Input: part model. Units: mm. Frame: model coordinates. A direction names the side the tool comes from. Round coordinates to 2 decimals unless told otherwise and drop trailing zeros. Loops run counter-clockwise (first coordinate to the right, second up) from the corner with the lowest first, then second, coordinate; pieces in that order, holes last. Notation, with made-up numbers: (18.5, -5.5) - (24.5, -5.5) arc R36 cw to (24.5, 33.5) - close; hole circle Ø4 at (50.5, -22.75). An arc over 180 degrees is marked (long way). One line per question, with ' | ' between items. Start each with the question number.
Item 1: First-contact query: pin 1 (13 mm diameter, centred on x = 11.5, y = 2.5, fed in from +Z); pin 2 (1.8 mm diameter, centred on x = -15.5, y = 17, fed in from -Z). Flat tips, straight axial feed; report the tip coordinate or a pass-through.
Item 2: Section B-B, the plane x = -15.5. Return loops of the section in (y, z), plus the area to 3 significant figures.
Item 3: Material intervals for line 1 along Y through (x, z) = (15.5, 2.5); line 2 along Y through (x, z) = (15.5, -1.8); line 3 along Y through (x, z) = (16, 33), sorted ascending.
Item 4: Set-up query: faces 4 (the face through (-17.07, -16.15, 2.46)), 5 (the face through (0, 0, 5)), 6 (the face through (-12.553, -15.63, -1.479)). Return all of +Z, -Z, +X, -X, +Y, -Y with unobstructed straight access to the full face (end or side cutting, diameter ignored); none if empty.
Item 5: Section D-D, the plane x = -3. Return loops of the section in (y, z).
Item 6: Section A-A, the plane y = -15.5. Return loops of the section in (x, z), plus the area to 3 significant figures.
Item 7: Section C-C, the plane z = 25. Return loops of the section in (x, y).
Item 8: Draft query along X for faces 1 (the face through (14, 14, 0)), 2 (the face through (26.5, 0, 0)), 3 (the face through (0, -24, 43)). Return one class per face: pulls with the +X half, pulls with the -X half, needs draft (parallel to the pull), parting line crosses it, or undercut.
```python
from build123d import *

# Parameters (mm, degrees)
SKETCH1_W           = 53
SKETCH1_H           = 43
BOSS_EXTRUDE1_DEPTH = 5
SKETCH2_W           = 53
SKETCH2_H           = 5
BOSS_EXTRUDE2_DEPTH = 43
SKETCH4_R           = 1.7
CUT_EXTRUDE1_DEPTH  = 58.039460025
SKETCH6_W           = 53
SKETCH6_H           = 53
SKETCH6_R           = 2.95
BOSS_EXTRUDE5_DEPTH = 3


with BuildPart() as part:
    # Sketch1 → Boss-Extrude1 (new body)
    with BuildSketch(Plane.XY):
        Rectangle(SKETCH1_W, SKETCH1_H)
    extrude(amount=BOSS_EXTRUDE1_DEPTH)

    # Sketch2 → Boss-Extrude2 (add)
    with BuildSketch(Plane(origin=(0, 0, 0), x_dir=(-1, 0, 0), z_dir=(0, 0, -1))):
        with Locations((0, -24)):
            Rectangle(SKETCH2_W, SKETCH2_H)
        with Locations((0, 24)):
            Rectangle(SKETCH2_W, SKETCH2_H)
    extrude(amount=-BOSS_EXTRUDE2_DEPTH)

    # Sketch4 → Cut-Extrude1 (cut, through all)
    with BuildSketch(Plane(origin=(0, 0, 0), x_dir=(-1, 0, 0), z_dir=(0, 0, -1))):
        with Locations((-15.5, 15.5)):
            Circle(SKETCH4_R)
        with Locations((15.5, 15.5)):
            Circle(SKETCH4_R)
        with Locations((-15.5, -15.5)):
            Circle(SKETCH4_R)
        with Locations((15.5, -15.5)):
            Circle(SKETCH4_R)
    extrude(amount=-CUT_EXTRUDE1_DEPTH, mode=Mode.SUBTRACT)

    # Sketch6 → Boss-Extrude5 (add)
    with BuildSketch(Plane.XY):
        Rectangle(SKETCH6_W, SKETCH6_H)
        with Locations((-15.5, 15.5)):
            Circle(SKETCH6_R, mode=Mode.SUBTRACT)
        with Locations(Location((15.5, 15.5, 0), (0, 0, 180))):
            Circle(SKETCH6_R, mode=Mode.SUBTRACT)
        with Locations(Location((-15.5, -15.5, 0), (0, 0, 180))):
            Circle(SKETCH6_R, mode=Mode.SUBTRACT)
        with Locations(Location((15.5, -15.5, 0), (0, 0, 180))):
            Circle(SKETCH6_R, mode=Mode.SUBTRACT)
    extrude(amount=-BOSS_EXTRUDE5_DEPTH)


solid = part.part
```
Return value:
1) pin 1: z = 5 | pin 2: z = 0
2) outline: (-26.5, -3) - (-18.45, -3) - (-18.45, 0) - (-17.2, 0) - (-17.2, 5) - (-21.5, 5) - (-21.5, 43) - (-26.5, 43) - close; (-13.8, 0) - (-12.55, 0) - (-12.55, -3) - (12.55, -3) - (12.55, 0) - (13.8, 0) - (13.8, 5) - (-13.8, 5) - close; (17.2, 0) - (18.45, 0) - (18.45, -3) - (26.5, -3) - (26.5, 43) - (21.5, 43) - (21.5, 5) - (17.2, 5) - close | area: 735 mm2
3) line 1: -26.5 to -17.2, -13.8 to 13.8, 17.2 to 26.5 | line 2: -26.5 to -18.45, -12.55 to 12.55, 18.45 to 26.5 | line 3: -26.5 to -21.5, 21.5 to 26.5
4) face 4: +Z, -Z | face 5: +Z, +X, -X | face 6: -Z
5) outline: (-26.5, -3) - (26.5, -3) - (26.5, 43) - (21.5, 43) - (21.5, 5) - (-21.5, 5) - (-21.5, 43) - (-26.5, 43) - close
6) outline: (-26.5, -3) - (-18.45, -3) - (-18.45, 0) - (-17.2, 0) - (-17.2, 5) - (-26.5, 5) - close; (-13.8, 0) - (-12.55, 0) - (-12.55, -3) - (12.55, -3) - (12.55, 0) - (13.8, 0) - (13.8, 5) - (-13.8, 5) - close; (17.2, 0) - (18.45, 0) - (18.45, -3) - (26.5, -3) - (26.5, 5) - (17.2, 5) - close | area: 355 mm2
7) outline: (-26.5, -26.5) - (26.5, -26.5) - (26.5, -21.5) - (-26.5, -21.5) - close; (-26.5, 21.5) - (26.5, 21.5) - (26.5, 26.5) - (-26.5, 26.5) - close
8) face 1: undercut | face 2: pulls with the +X half | face 3: needs draft
